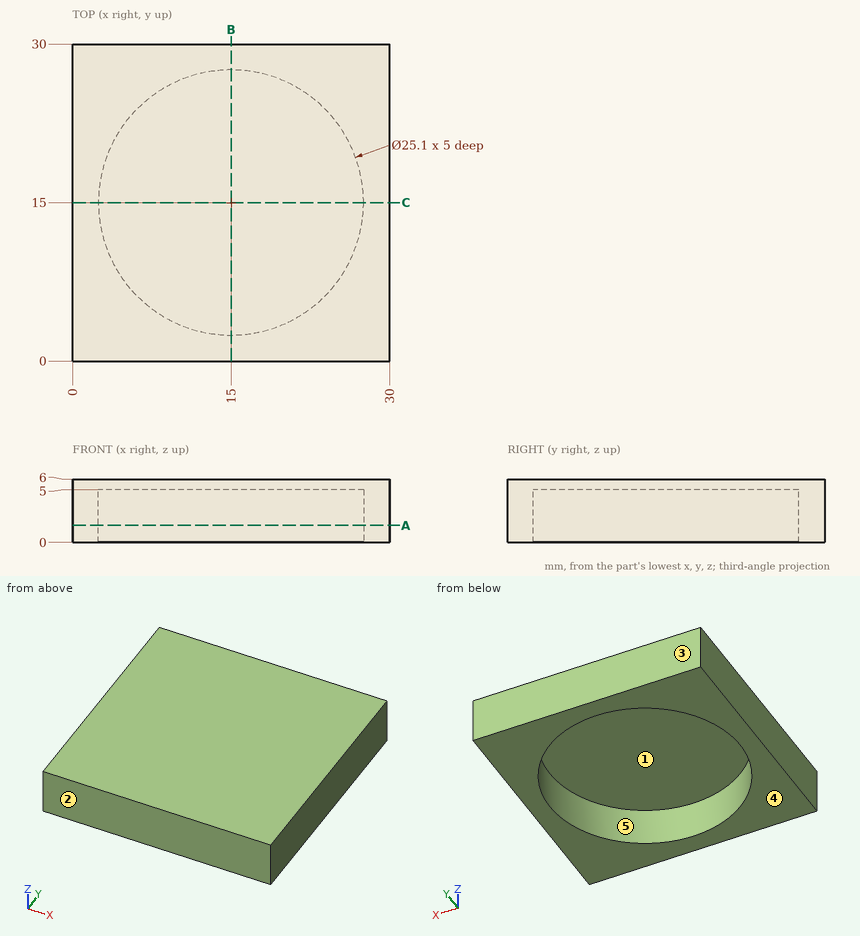
Geometry: see drawing. Coordinates: mm, zero at the bounding-box minimum. A direction names the side the tool comes from. Give positions to 0.01 mm unless a question says otherwise; leave off trailing zeros. Write each loop counter-clockwise with the first axis right and the second up, starting at its lowest first coordinate (ties: lowest second). Pieces come first, ordered by that corner, then holes. Notation, with made-up numbers: M 54.25,49.5 L 109.25,49.5 A31 cw 109.25,76.5 Z; hole C 88.25,-31.5 d5. An arc over 180 degrees is marked long. Return JSON: item names as keys, results as strings. Group by question number.
1) Cut plane B-B, the plane x = 15. Output: boundary loops of the cut face in (y, z).
2) Cut plane A-A, the plane z = 1.6. Output: boundary loops of the cut face in (x, y), then the cut area to 3 significant figures.
3) Ray query, L1, parallel to Y at x = 15, z = 3.7; L2, parallel to Z at x = 11.25, y = 17; L3, parallel to X at y = 10, z = 2.1. Return the intervals inside material, ascending.
4) Draft query along Y for the marked faces 3, 4 and 5. Return one class per face: released by +Y, released by -Y, zero draft, split by the parting line, or undercut.
5) First-contact query: pin 1 Ø7.5 at (x, y) = (13.5, 9.5) entering from -Z; pin 2 Ø1 at (x, z) = (11.5, 2) entering from -Y. Flat tips, straight axial feed; report the tip coordinate or a pass-through.
6) Set-up query: the marked faces 1 and 2. Return all of +Z, -Z, +X, -X, +Y, -Y with unobstructed straight access to the full face (end or side cutting, diameter ignored); none if empty.
Data:
{
 "1": {"outline": "M 0,0 L 2.45,0 L 2.45,5 L 27.55,5 L 27.55,0 L 30,0 L 30,6 L 0,6 Z"},
 "2": {"outline": "M 0,0 L 30,0 L 30,30 L 0,30 Z; hole C 15,15 d25.1", "area": "405 mm²"},
 "3": {"L1": "y = 0 to 2.45, 27.55 to 30", "L2": "z = 5 to 6", "L3": "x = 0 to 3.49, 26.51 to 30"},
 "4": {"face 3": "released by +Y", "face 4": "zero draft", "face 5": "undercut"},
 "5": {"pin 1": "stops at z = 5", "pin 2": "stops at y = 0"},
 "6": {"face 1": "-Z", "face 2": "+Z, -Z, +X, -X, -Y"}
}
